Geometry check sheet. Reference: the model listing, model coordinates, mm. A direction names the side the tool comes from. Coordinates: 2 decimals unless noted, no trailing zeros. Write each loop counter-clockwise with the first axis right and the second up, starting at its lowest first coordinate (ties: lowest second). Pieces come first, ordered by that corner, then holes. Notation, with made-up numbers: (77, 84) -> (123, 84) arc R24 cw to (123, 110) -> close; hole circle Ø7 at (33, 34). An arc over 180 degrees is marked (long way). Answer in a Markdown table with one row per item. Add a question column.
1. Cross-section at B-B on x = 7.62. Record the cut outline in (y, z), and give its area (3 significant figures).
2. Set-up check for faces 1 (the flat face through (1, 6.4, 1.9)), 2 (the flat face through (4, 6, 0)), 3 (the cylindrical face through (1.905, 6.042, 3.246)), 4 (the flat face through (14.24, 4.6, 1.9)), 5 (the cylindrical face through (13.37, 5.54, 3.43)): record each of +Z, -Z, +X, -X, +Y, -Y from which the full face is reachable in a straight line by a thin tool's end or side.
3. Cross-section at D-D on y = 3.25. Record the cut outline in (x, z).
4. Mould release check, pull along Y, two halves, no side actions. Record for faces 6 (the cylindrical face through (14.428, 8.744, 2.504)), 7 (the flat face through (8, 0, 1)), 8 (the flat face through (0, 10, 3)): pulls with the +Y half, pulls with the -Y half, needs draft (parallel to the pull), parting line crosses it, or undercut.
5. Cross-section at A-A on y = 5.5. Record the cut outline in (x, z), and give its area (3 significant figures).
6. Depth check by flat-ended pin: P1, Ø5.5, axis at x = 7.62, y = 5.5, coming from the +Z side; P2, Ø1.6, axis at y = 5.5, z = 2.54, coming from the +X side; P3, Ø3, axis at y = 6, z = 2, coming from the +X side; P4, Ø2, axis at y = 5.5, z = 2.54, coming from the -X side. Enter the tip coordinate at first touch or a pass-through.
7. Scan lines: L1, parallel to Z at x = 1.65, y = 5.5; L2, parallel to X at y = 8, z = 4.8; L3, parallel to Y at x = 7.62, z = 2.8. Record each from-to range of solid material in increasing order. Write a range as from..to.
8. Cross-section at C-C on z = 0.4. Give the number of separate pieces and of enclosed holes in the cut face, and give its area (3 significant figures).
```python
from build123d import *

# Parameters (mm, degrees)
SKETCH1_R           = 0.8509
SKETCH1_R_2         = 3.4925
BOSS_EXTRUDE1_DEPTH = 5.08
SKETCH2_R           = 0.89
CUT_EXTRUDE1_DEPTH  = 2.286
CUT_EXTRUDE2_START  = -2.286
SKETCH3_R           = 0.89
CUT_EXTRUDE2_DEPTH  = 2.286
CUT_EXTRUDE3_DEPTH  = 20.46956602


with BuildPart() as part:
    # Sketch1 → Boss-Extrude1 (new body)
    with BuildSketch(Plane.XY):
        with BuildLine():
            ThreePointArc((0, 9.75), (0.804883509, 8.760503782), (1, 7.5))
            Line((1, 7.5), (1, 3.5))
            ThreePointArc((1, 3.5), (0.804883509, 2.239496218), (0, 1.25))
            Line((0, 1.25), (0, 0))
            Line((0, 0), (15.24, 0))
            Line((15.24, 0), (15.24, 1.25))
            ThreePointArc((15.24, 1.25), (14.435116491, 2.239496218), (14.24, 3.5))
            Line((14.24, 3.5), (14.24, 7.5))
            ThreePointArc((14.24, 7.5), (14.435116491, 8.760503782), (15.24, 9.75))
            Line((15.24, 9.75), (15.24, 11))
            Line((15.24, 11), (0, 11))
            Line((0, 11), (0, 9.75))
        make_face()
        with Locations((2.886809291, 5.5)):
            Circle(SKETCH1_R, mode=Mode.SUBTRACT)
        with Locations((7.62, 5.5)):
            Circle(SKETCH1_R_2, mode=Mode.SUBTRACT)
        with Locations((12.353190709, 5.5)):
            Circle(SKETCH1_R, mode=Mode.SUBTRACT)
    extrude(amount=BOSS_EXTRUDE1_DEPTH)

    # Sketch2 → Cut-Extrude1 (cut)
    with BuildSketch(Plane(origin=(14.24, 0, 0), x_dir=(0, 0, -1), z_dir=(1, 0, 0))):
        with Locations((-2.54, 5.5)):
            Circle(SKETCH2_R)
    extrude(amount=-CUT_EXTRUDE1_DEPTH, mode=Mode.SUBTRACT)

    # Sketch3 → Cut-Extrude2 (cut)
    with BuildSketch(Plane.ZY.offset(-1).offset(CUT_EXTRUDE2_START)):
        with Locations(Location((2.54, 5.5, 0), (0, 0, 180))):
            Circle(SKETCH3_R)
    extrude(amount=CUT_EXTRUDE2_DEPTH, mode=Mode.SUBTRACT)

    # Sketch4 → Cut-Extrude3 (cut, through all)
    with BuildSketch(Plane(origin=(15.24, 0, 0), x_dir=(0, 0, -1), z_dir=(1, 0, 0))):
        with BuildLine():
            Line((-2.94, 0), (-2.14, 0))
            Line((-2.14, 0), (-2.14, 0.376))
            ThreePointArc((-2.14, 0.376), (-2.249542064, 0.640457936), (-2.514, 0.75))
            Line((-2.514, 0.75), (-2.566, 0.75))
            ThreePointArc((-2.566, 0.75), (-2.830457936, 0.640457936), (-2.94, 0.376))
            Line((-2.94, 0.376), (-2.94, 0))
        make_face()
    cut_extrude3 = extrude(amount=-CUT_EXTRUDE3_DEPTH, mode=Mode.SUBTRACT)

    # Mirror1: Cut-Extrude3 across plane
    add(cut_extrude3.mirror(Plane(origin=(0, 5.5, 0), x_dir=(0, 0, 1), z_dir=(0, -1, 0))), mode=Mode.SUBTRACT)


solid = part.part
```
Results found:
| question | item | result |
|---|---|---|
| 1 | outline | (0, 0) -> (2.01, 0) -> (2.01, 5.08) -> (0, 5.08) -> (0, 2.94) -> (0.38, 2.94) arc R0.37 cw to (0.75, 2.57) -> (0.75, 2.51) arc R0.37 cw to (0.38, 2.14) -> (0, 2.14) -> close; (8.99, 0) -> (11, 0) -> (11, 2.14) -> (10.62, 2.14) arc R0.37 cw to (10.25, 2.51) -> (10.25, 2.57) arc R0.37 cw to (10.62, 2.94) -> (11, 2.94) -> (11, 5.08) -> (8.99, 5.08) -> close |
| 1 | area | 19.3 mm^2 |
| 2 | face 1 | +Z, -Z, -X |
| 2 | face 2 | -Z, +X, -X, +Y, -Y |
| 2 | face 3 | -X |
| 2 | face 4 | +Z, -Z, +X |
| 2 | face 5 | +X |
| 3 | outline | (1.01, 0) -> (4.95, 0) -> (4.95, 5.08) -> (1.01, 5.08) -> close; (10.29, 0) -> (14.23, 0) -> (14.23, 5.08) -> (10.29, 5.08) -> close |
| 4 | face 6 | undercut |
| 4 | face 7 | pulls with the -Y half |
| 4 | face 8 | needs draft |
| 5 | outline | (1, 0) -> (2.04, 0) -> (2.04, 1.65) -> (1, 1.65) -> close; (1, 3.43) -> (2.04, 3.43) -> (2.04, 5.08) -> (1, 5.08) -> close; (3.74, 0) -> (4.13, 0) -> (4.13, 5.08) -> (3.74, 5.08) -> close; (11.11, 0) -> (11.5, 0) -> (11.5, 5.08) -> (11.11, 5.08) -> close; (13.2, 0) -> (14.24, 0) -> (14.24, 1.65) -> (13.2, 1.65) -> close; (13.2, 3.43) -> (14.24, 3.43) -> (14.24, 5.08) -> (13.2, 5.08) -> close |
| 5 | area | 10.8 mm^2 |
| 6 | P1 | passes through |
| 6 | P2 | stops at x = 11.95 |
| 6 | P3 | stops at x = 14.24 |
| 6 | P4 | stops at x = 1 |
| 7 | L1 | z = 0..1.65, 3.43..5.08 |
| 7 | L2 | x = 1..5.18, 10.06..14.24 |
| 7 | L3 | y = 0.67..2.01, 8.99..10.33 |
| 8 | separate pieces | 1 |
| 8 | enclosed holes | 3 |
| 8 | area | 110 mm^2 |
